Drawing for the job (mm, zero at the part's lowest x, y, z). A direction names the side the tool comes from. Coordinates: 2 decimals unless noted, no trailing zeros. Write each loop counter-clockwise with the first axis right and the second up, starting at its lowest first coordinate (ties: lowest second). Pieces come first, ordered by that corner, then holes. Notation, with made-up numbers: M -14,-15.5 L 12,-15.5 A26 cw 12,10.5 Z; hole C -29,-21.75 d3. An arc over 180 degrees is marked long. Use CSV: the item, a comma, the result in double quotes. Start each with the question number.
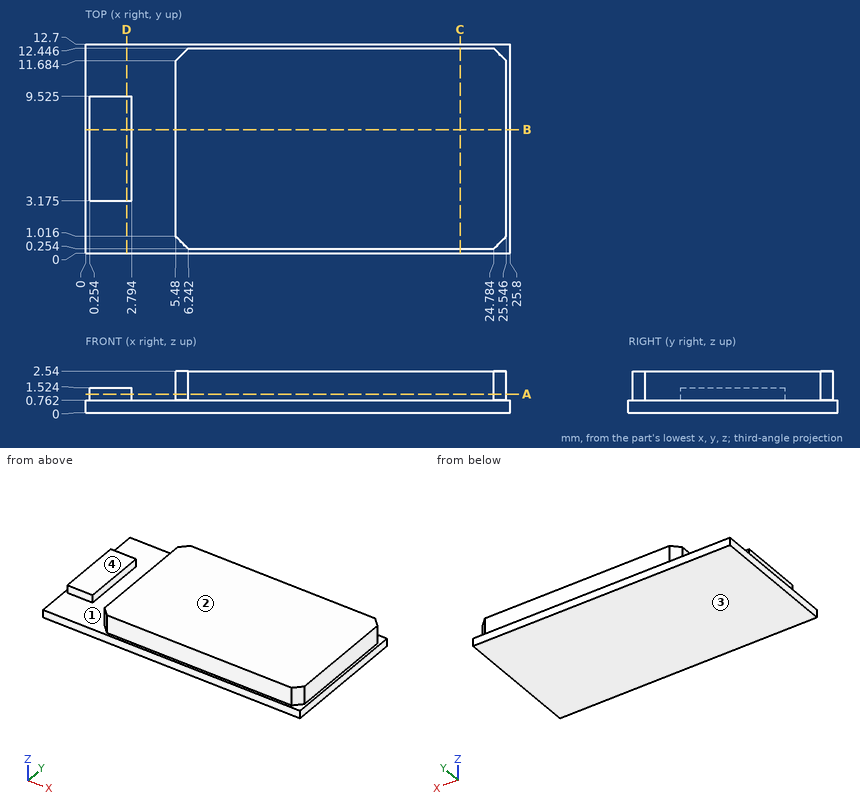
1) Band-saw the part on C-C on x = 22.75. List the corners of the cut face in (y, z), then the cut area to 3 significant figures.
2) Band-saw the part on A-A on z = 1.15. List the corners of the cut face in (x, y) (3 decimals), then the cut area to 3 significant figures.
3) Band-saw the part on D-D on x = 2.5. List the corners of the cut face in (y, z) (3 decimals).
4) Tool access for the marked faces 3 and 4: list every direction of +Z, -Z, +X, -X, +Y, -Y with a clear straight run to the whole face (end or side of a thin tool).
5) Drop flat-ended pins along their axis: P1, Ø0.5, axis at x = 18, z = 2, coming from the +Y side; P2, Ø0.5, axis at y = 7.5, z = 1.5, coming from the -X side; P3, Ø1.3, axis at x = 1.5, y = 6.5, coming from the +Z side. Give the stop position or say it passes through.
6) Band-saw the part on B-B on y = 7.5. List the corners of the cut face in (x, z), then the cut area to 3 significant figures.
7) Wall check: L1, parallel to X at y = 8.75, z = 1.4; L2, parallel to Y at x = 18.5, z = 2.1; L3, parallel to Y at x = 1.5, z = 1.15 (3 decimals). Give the ranges that are in metal, low to high. Write a range as [from, to].
8) Two-plate mould, pull along X, no slides. Class the marked faces 1 and 2: pulls with the +X half, pulls with the -X half, needs draft (parallel to the pull), parting line crosses it, or undercut.
Findings below:
1,outline,"M 0,0 L 12.7,0 L 12.7,0.76 L 12.45,0.76 L 12.45,2.54 L 0.25,2.54 L 0.25,0.76 L 0,0.76 Z"
1,area,"31.4 mm2"
2,outline,"M 0.254,3.175 L 2.794,3.175 L 2.794,9.525 L 0.254,9.525 Z; M 5.48,1.016 L 6.242,0.254 L 24.784,0.254 L 25.546,1.016 L 25.546,11.684 L 24.784,12.446 L 6.242,12.446 L 5.48,11.684 Z"
2,area,"260 mm2"
3,outline,"M 0,0 L 12.7,0 L 12.7,0.762 L 9.525,0.762 L 9.525,1.524 L 3.175,1.524 L 3.175,0.762 L 0,0.762 Z"
4,face 3,"-Z, +X, -X, +Y, -Y"
4,face 4,"+Z, -X, +Y, -Y"
5,P1,"stops at y = 12.45"
5,P2,"stops at x = 0.25"
5,P3,"stops at z = 1.52"
6,outline,"M 0,0 L 25.8,0 L 25.8,0.76 L 25.55,0.76 L 25.55,2.54 L 5.48,2.54 L 5.48,0.76 L 2.79,0.76 L 2.79,1.52 L 0.25,1.52 L 0.25,0.76 L 0,0.76 Z"
6,area,"57.3 mm2"
7,L1,"x = [0.25, 2.79], [5.48, 25.55]"
7,L2,"y = [0.25, 12.45]"
7,L3,"y = [3.175, 9.525]"
8,face 1,"undercut"
8,face 2,"needs draft"
